Part model, mm, in its own coordinate system. A direction names the side the tool comes from. Give positions to 0.01 mm unless a question says otherwise; leave off trailing zeros. Write each loop counter-clockwise with the first axis right and the second up, starting at its lowest first coordinate (ties: lowest second). Pieces come first, ordered by that corner, then holes. Notation, with made-up numbers: M 7,36.25 L 14,36.25 A13 ccw 14,47.25 Z; hole C -8.5,89 d5. An arc over 180 degrees is marked long. Answer as CSV lines item,"result". Start each with the question number.
1) Pin check, flat tips, straight feed: pin 1 Ø2 at (y, z) = (-31, 1) entering from -X; pin 2 Ø3 at (x, y) = (8, -73.5) entering from +Z. Stop position of each tip, or through.
2) Slice it at A-A, the plane y = 5. Give the cut face in (x, z), plus the area to 3 significant figures.
3) Slice it at B-B, the plane x = 3.75. Give the cut face in (y, z).
4) Wall check: line 1 along Y through (x, z) = (5, 6.5); line 2 along Y through (x, z) = (8.5, 8.25); line 3 along Y through (x, z) = (1, 8.5). Give the ranges that are in metal, low to high. Write a range as from..to.
5) Slice it at C-C, the plane x = 9. Give the cut face in (y, z).
6) Tool access for faces 4 (the cylindrical face through (0.12, -39.44, 6.08)), 5 (the flat face through (3, 7, 10)), 6 (the flat face through (9, 0, 1)), 7 (the flat face through (1, 0, 1)), 8 (the flat face through (9, 0, 9)): list every direction of +Z, -Z, +X, -X, +Y, -Y with a clear straight run to the whole face (end or side of a thin tool).
7) Slice it at D-D, the plane z = 6. Give the cut face in (x, y), plus the area to 3 significant figures.
8) Mould opens along Y. For faces 1 (the flat face through (10, 5, 5)), 2 (the cylindrical face through (7.385, 5.751, 5.07)), 3 (the flat face through (1, 0, 9)) say: pulls with the +Y half, pulls with the -Y half, needs draft (parallel to the pull), parting line crosses it, or undercut.
```python
from build123d import *

# Parameters (mm, degrees)
SKETCH2_W           = 10
SKETCH2_H           = 10
BOSS_EXTRUDE2_DEPTH = 10
SKETCH5_R           = 2.5
CUT_EXTRUDE1_DEPTH  = 10
SKETCH6_R           = 5
BOSS_EXTRUDE4_DEPTH = 80
SKETCH7_R           = 3
BOSS_EXTRUDE5_DEPTH = 7


with BuildPart() as part:
    # Sketch2 → Boss-Extrude2 (new body)
    with BuildSketch(Plane.XY):
        with Locations((5, 5)):
            Rectangle(SKETCH2_W, SKETCH2_H)
    extrude(amount=BOSS_EXTRUDE2_DEPTH)

    # Sketch5 → Cut-Extrude1 (cut)
    with BuildSketch(Plane.XY.offset(10)):
        with Locations((5, 5)):
            Circle(SKETCH5_R)
    extrude(amount=-CUT_EXTRUDE1_DEPTH, mode=Mode.SUBTRACT)

    # Sketch6 → Boss-Extrude4 (add)
    with BuildSketch(Plane.XZ):
        with Locations(Location((5, 5, 0), (0, 0, 270))):
            Circle(SKETCH6_R)
    extrude(amount=BOSS_EXTRUDE4_DEPTH)

    # Sketch7 → Boss-Extrude5 (add)
    with BuildSketch(Plane.XZ.offset(80)):
        with Locations(Location((5, 5, 0), (0, 0, 270))):
            Circle(SKETCH7_R)
    extrude(amount=BOSS_EXTRUDE5_DEPTH)


solid = part.part
```
Found:
1,pin 1,"x = 1"
1,pin 2,"z = 9.77"
2,outline,"M 0,0 L 2.5,0 L 2.5,10 L 0,10 Z; M 7.5,0 L 10,0 L 10,10 L 7.5,10 Z"
2,area,"50.0 mm²"
3,outline,"M -87,2.27 L -80,2.27 L -80,0.16 L 0,0.16 L 0,0 L 2.83,0 L 2.83,10 L 0,10 L 0,9.84 L -80,9.84 L -80,7.73 L -87,7.73 Z; M 7.17,0 L 10,0 L 10,10 L 7.17,10 Z"
4,line 1,"-87..2.5, 7.5..10"
4,line 2,"-80..10"
4,line 3,"0..10"
5,outline,"M -80,2 L 0,2 L 0,0 L 10,0 L 10,10 L 0,10 L 0,8 L -80,8 Z"
6,face 4,"-Y"
6,face 5,"+Z, +X, -X, +Y, -Y"
6,face 6,"-Z, +X, -Y"
6,face 7,"-Z, -X, -Y"
6,face 8,"+Z, +X, -Y"
7,outline,"M 0,0 L 0.1,0 L 0.1,-80 L 2.17,-80 L 2.17,-87 L 7.83,-87 L 7.83,-80 L 9.9,-80 L 9.9,0 L 10,0 L 10,10 L 0,10 Z; hole C 5,5 d5"
7,area,"904 mm²"
8,face 1,"needs draft"
8,face 2,"undercut"
8,face 3,"pulls with the -Y half"
